Source: CAD feature listing. Evaluate the final solid. Frame: model axes, mm. A direction names the side the tool comes from. Round coordinates to 2 decimals unless told otherwise and drop trailing zeros. Order: outer loops, then holes, each group sorted by start corner. A loop starts at its lowest first (then second) coordinate and runs counter-clockwise, first axis right, second up. Notation, with made-up numbers: (-29.5, 63) - (-20.5, 63) arc R12 ccw to (-20.5, 67) - close; hole circle Ø4 at (37.5, -23.5). An arc over 180 degrees is marked (long way). Put each result on its own line as item: value. Start each with the question number.
1) Access query for faces 4 (the face through (7, -5, -13)), 5 (the face through (-8.5, -5, 13)), 6 (the face through (-2.832, -5, -12.5)), 7 (the face through (4.4, -5, 12)), 8 (the face through (21, -1, -12)). Directions: +Z, -Z, +X, -X, +Y, -Y. A direction counts if a zero-diameter tool reaches every point of the face in a straight line with its end or side. Return the directions, or none.
2) Mould query, pull axis X, two halves, no side actions, for faces 1 (the face through (1.352, -5, 12.5)), 2 (the face through (20.5, -5, -12.5)), 3 (the face through (4.4, -5, -12)). Classes: +X half, -X half, draft (parallel to the pull), parting line (faces both ways), or undercut.
3) Section C-C on y = -7. State how many separate pieces and enclosed holes the cut face has, then the cut area to 3 significant figures.
4) Section A-A on x = -23.5. Output: boundary loops of the cut face in (y, z).
5) Section B-B on z = -1.75. Output: boundary loops of the cut face in (x, y).
6) Contact query for flat-ended pins moving along their axis: P1, Ø0.5, axis at x = 20, y = -5.5, coming from the -Z side; P2, Ø0.8, axis at y = -5.5, z = -12.5, coming from the -X side (3 decimals); P3, Ø0.8, axis at x = -0.5, y = -6, coming from the +Z side. Output: stop coordinate, or through.
7) Line query: probe 1 along X at (y, z) = (0.9, -12.25); probe 2 along Z at (x, y) = (-2, -1.5); probe 3 along Z at (x, y) = (7.5, -6.5). Output: solid intervals per line, ascending. Write a range as [from, to].
```python
from build123d import *

# Parameters (mm, degrees)
SKETCH1_R           = 1.5
BOSS_EXTRUDE1_DEPTH = 1.5
SKETCH2_W           = 38.5
SKETCH2_H           = 2
BOSS_EXTRUDE2_DEPTH = 2
SKETCH3_W           = 17.5
SKETCH3_H           = 16
BOSS_EXTRUDE3_DEPTH = 3
SKETCH4_W           = 1
SKETCH4_H           = 1
BOSS_EXTRUDE4_DEPTH = 8


with BuildPart() as part:
    # Sketch1 → Boss-Extrude1 (new body)
    with BuildSketch(Plane(origin=(0, 0, 0), x_dir=(1, 0, 0), z_dir=(0, 1, 0))):
        with BuildLine():
            Line((24, -14.5), (-24, -14.5))
            ThreePointArc((-24, -14.5), (-25.414213562, -13.914213562), (-26, -12.5))
            Line((-26, -12.5), (-26, 12.5))
            ThreePointArc((-26, 12.5), (-25.414213562, 13.914213562), (-24, 14.5))
            Line((-24, 14.5), (24, 14.5))
            ThreePointArc((24, 14.5), (25.414213562, 13.914213562), (26, 12.5))
            Line((26, 12.5), (26, -12.5))
            ThreePointArc((26, -12.5), (25.414213562, -13.914213562), (24, -14.5))
        make_face()
        with Locations(Location((-23.5, 12.25, 0), (0, 0, 270))):
            Circle(SKETCH1_R, mode=Mode.SUBTRACT)
        with Locations(Location((23.5, 12.25, 0), (0, 0, 90))):
            Circle(SKETCH1_R, mode=Mode.SUBTRACT)
        with Locations(Location((23.5, -12.25, 0), (0, 0, 270))):
            Circle(SKETCH1_R, mode=Mode.SUBTRACT)
        with Locations(Location((-23.5, -12.25, 0), (0, 0, 90))):
            Circle(SKETCH1_R, mode=Mode.SUBTRACT)
    extrude(amount=BOSS_EXTRUDE1_DEPTH)

    # Sketch2 → Boss-Extrude2 (add)
    with BuildSketch(Plane(origin=(0, 0, 0), x_dir=(1, 0, 0), z_dir=(0, 1, 0))):
        with Locations((1.75, -12.5)):
            Rectangle(SKETCH2_W, SKETCH2_H)
        with Locations((1.75, 12.5)):
            Rectangle(SKETCH2_W, SKETCH2_H)
    extrude(amount=-BOSS_EXTRUDE2_DEPTH)

    # Sketch3 → Boss-Extrude3 (add)
    with BuildSketch(Plane(origin=(0, 1.5, 0), x_dir=(1, 0, 0), z_dir=(0, 1, 0))):
        with Locations((10.25, 0)):
            Rectangle(SKETCH3_W, SKETCH3_H)
    extrude(amount=BOSS_EXTRUDE3_DEPTH)

    # Sketch4 → Boss-Extrude4 (add)
    with BuildSketch(Plane(origin=(0, 0, 0), x_dir=(1, 0, 0), z_dir=(0, 1, 0))):
        with Locations((20, 12.5)):
            Rectangle(SKETCH4_W, SKETCH4_H)
        with Locations((17.4075, 12.5)):
            Rectangle(SKETCH4_W, SKETCH4_H)
        with Locations((14.815, 12.5)):
            Rectangle(SKETCH4_W, SKETCH4_H)
        with Locations((12.2225, 12.5)):
            Rectangle(SKETCH4_W, SKETCH4_H)
        with Locations((9.63, 12.5)):
            Rectangle(SKETCH4_W, SKETCH4_H)
        with Locations((7.0375, 12.5)):
            Rectangle(SKETCH4_W, SKETCH4_H)
        with Locations((4.445, 12.5)):
            Rectangle(SKETCH4_W, SKETCH4_H)
        with Locations((1.8525, 12.5)):
            Rectangle(SKETCH4_W, SKETCH4_H)
        with Locations((-0.74, 12.5)):
            Rectangle(SKETCH4_W, SKETCH4_H)
        with Locations((-3.3325, 12.5)):
            Rectangle(SKETCH4_W, SKETCH4_H)
        with Locations((-5.925, 12.5)):
            Rectangle(SKETCH4_W, SKETCH4_H)
        with Locations((-8.5175, 12.5)):
            Rectangle(SKETCH4_W, SKETCH4_H)
        with Locations((-11.11, 12.5)):
            Rectangle(SKETCH4_W, SKETCH4_H)
        with Locations((-13.7025, 12.5)):
            Rectangle(SKETCH4_W, SKETCH4_H)
        with Locations((-16.295, 12.5)):
            Rectangle(SKETCH4_W, SKETCH4_H)
        with Locations((-16.295, -12.5)):
            Rectangle(SKETCH4_W, SKETCH4_H)
        with Locations((-13.7025, -12.5)):
            Rectangle(SKETCH4_W, SKETCH4_H)
        with Locations((-11.11, -12.5)):
            Rectangle(SKETCH4_W, SKETCH4_H)
        with Locations((-8.5175, -12.5)):
            Rectangle(SKETCH4_W, SKETCH4_H)
        with Locations((-5.925, -12.5)):
            Rectangle(SKETCH4_W, SKETCH4_H)
        with Locations((-3.3325, -12.5)):
            Rectangle(SKETCH4_W, SKETCH4_H)
        with Locations((-0.74, -12.5)):
            Rectangle(SKETCH4_W, SKETCH4_H)
        with Locations((1.8525, -12.5)):
            Rectangle(SKETCH4_W, SKETCH4_H)
        with Locations((4.445, -12.5)):
            Rectangle(SKETCH4_W, SKETCH4_H)
        with Locations((7.0375, -12.5)):
            Rectangle(SKETCH4_W, SKETCH4_H)
        with Locations((9.63, -12.5)):
            Rectangle(SKETCH4_W, SKETCH4_H)
        with Locations((12.2225, -12.5)):
            Rectangle(SKETCH4_W, SKETCH4_H)
        with Locations((14.815, -12.5)):
            Rectangle(SKETCH4_W, SKETCH4_H)
        with Locations((17.4075, -12.5)):
            Rectangle(SKETCH4_W, SKETCH4_H)
        with Locations((20, -12.5)):
            Rectangle(SKETCH4_W, SKETCH4_H)
    extrude(amount=-BOSS_EXTRUDE4_DEPTH)


solid = part.part
```
Answer sheet:
1. face 4: -Z, +X, -X, -Y
1. face 5: +Z, +X, -X, -Y
1. face 6: +Z, -Z, -Y
1. face 7: +X, -X, -Y
1. face 8: +Z, -Z, +X, -Y
2. face 1: undercut
2. face 2: +X half
2. face 3: draft
3. separate pieces: 30
3. enclosed holes: 0
3. area: 30.0 mm^2
4. outline: (0, -14.5) - (1.5, -14.5) - (1.5, -13.75) - (0, -13.75) - close; (0, -10.75) - (1.5, -10.75) - (1.5, 10.75) - (0, 10.75) - close; (0, 13.75) - (1.5, 13.75) - (1.5, 14.5) - (0, 14.5) - close
5. outline: (-26, 0) - (26, 0) - (26, 1.5) - (19, 1.5) - (19, 4.5) - (1.5, 4.5) - (1.5, 1.5) - (-26, 1.5) - close
6. P1: z = -13
6. P2: x = -16.795
6. P3: z = 13
7. probe 1: [-26, -25], [-22, 22], [25, 26]
7. probe 2: [-13.5, -11.5], [11.5, 13.5]
7. probe 3: [-13, -12], [12, 13]
